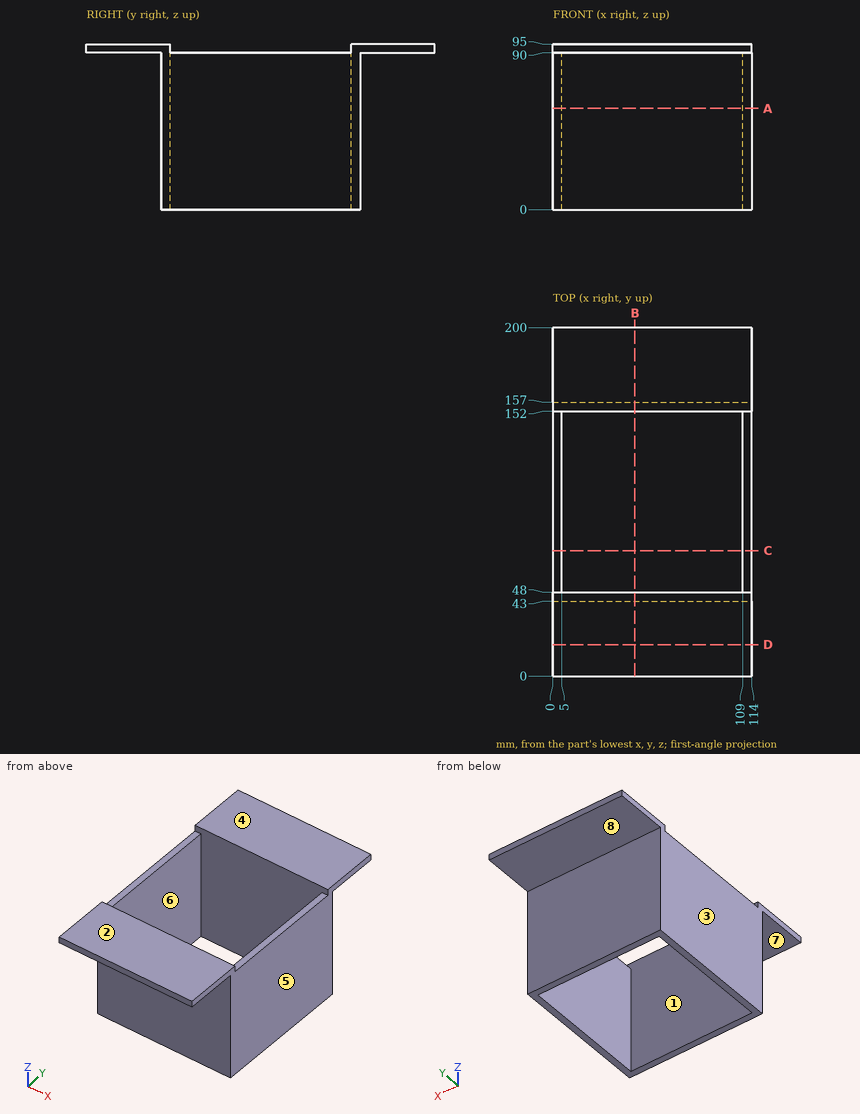
Answer from the drawing. Dimensions are ordinates in mm from the lowest x, y and z of the part. A direction names the side the tool comes from. Round coordinates to 2 decimals unless told otherwise and drop trailing zeros. Order: outer loops, then holes, each group sorted by start corner. A loop starts at its lowest first (then second) coordinate and runs counter-clockwise, first axis right, second up.
1) Flat-ended cylindrical pins translate along their axes: pin 1 (4 mm diameter, centred on y = 90.5, z = 34.5, fed in from -X); pin 2 (1.5 mm diameter, centred on x = 102.5, z = 44.5, fed in from +Y); pin 3 (5.5 mm diameter, centred on x = 3, y = 83, fed in from +Z); pin 4 (3 mm diameter, centred on x = 51.5, z = 41, fed in from -Y). Find the tip coordinate at first contact, or state that the pin passes through.
2) The part is cut by section C-C on y = 72. Write down the section's boundary in (x, z), plus the area to 3 significant figures.
3) The mould has two halves that part along X. Classify the marked faces 1, 2 and 3: released by +X, released by -X, zero draft, split by the parting line, or undercut.
4) The part is cut by section A-A on z = 58. Write down the section's boundary in (x, y).
5) For the marked faces 4, 5, 6, 7 and 8, determine the directions among +Z, -Z, +X, -X, +Y, -Y from which every point of the face is accessible in a straight line to the end or side of a thin tool.
6) Straight lines are drawn through the part: L1, parallel to Y at x = 84, z = 5; L2, parallel to X at y = 78.5, z = 11.5; L3, parallel to Z at x = 88, y = 164. For each, find the intervals that lie inside material, in ascending order.
7) The part is cut by section D-D on y = 18. Write down the section's boundary in (x, z), plus the area to 3 significant figures.
8) The part is cut by section B-B on x = 47. Write down the section's boundary in (y, z), plus the area to 3 significant figures.
Resolved:
1. pin 1: stops at x = 0
1. pin 2: stops at y = 157
1. pin 3: stops at z = 90
1. pin 4: stops at y = 43
2. outline: (0, 0) - (5, 0) - (5, 90) - (0, 90) - close; (109, 0) - (114, 0) - (114, 90) - (109, 90) - close
2. area: 900 mm2
3. face 1: undercut
3. face 2: zero draft
3. face 3: released by -X
4. outline: (0, 43) - (114, 43) - (114, 157) - (0, 157) - close; hole (5, 48) - (109, 48) - (109, 152) - (5, 152) - close
5. face 4: +Z, +X, -X, +Y, -Y
5. face 5: +Z, -Z, +X, +Y, -Y
5. face 6: +Z, -Z
5. face 7: -Z, +X, -X, -Y
5. face 8: -Z, +X, -X, +Y
6. L1: y = 43 to 48, 152 to 157
6. L2: x = 0 to 5, 109 to 114
6. L3: z = 90 to 95
7. outline: (0, 90) - (114, 90) - (114, 95) - (0, 95) - close
7. area: 570 mm2
8. outline: (0, 90) - (43, 90) - (43, 0) - (48, 0) - (48, 95) - (0, 95) - close; (152, 0) - (157, 0) - (157, 90) - (200, 90) - (200, 95) - (152, 95) - close
8. area: 1,380 mm2
